Can you work these out from the model? Positions are in its coordinate system, mm. A direction names the side the tool comes from. Coordinates: 2 decimals unless noted, no trailing zeros. Write each loop counter-clockwise with the first axis right and the second up, starting at its lowest first coordinate (ties: lowest second). Pieces come first, ordered by that corner, then holes. Notation, with made-up numbers: (-26.75, 79) - (-2.75, 79) arc R10 cw to (-2.75, 84) - close; hole circle Ø8 at (7.5, 52). An arc over 180 degrees is marked (long way). One line per question, with ' | ' between items. Start each with the question number.
from build123d import *

# Parameters (mm, degrees)
F0_R     = 25
F0_R_2   = 15
F1_DEPTH = 28
F2_DEPTH = 116
F3_DEPTH = 28.5
F4_DEPTH = 50.8


with BuildPart() as f1:
    # F0 (on Top) → F1 (new body)
    with BuildSketch(Plane.XY):
        with BuildLine():
            Line((0, -44.5), (44.5, -44.5))
            Line((44.5, -44.5), (44.5, 0))
            ThreePointArc((44.5, 0), (31.466252, -31.466252), (0, -44.5))
        make_face()
        with BuildLine():
            Line((-44.5, -44.5), (0, -44.5))
            ThreePointArc((0, -44.5), (-31.466252, -31.466252), (-44.5, 0))
            Line((-44.5, 0), (-44.5, -44.5))
        make_face()
        with BuildLine():
            ThreePointArc((0, 44.5), (31.466252, 31.466252), (44.5, 0))
            Line((44.5, 0), (44.5, 44.5))
            Line((44.5, 44.5), (0, 44.5))
        make_face()
        with BuildLine():
            Line((-44.5, 44.5), (-44.5, 0))
            ThreePointArc((-44.5, 0), (-31.466252, 31.466252), (0, 44.5))
            Line((0, 44.5), (-44.5, 44.5))
        make_face()
        Circle(F0_R)
        Circle(F0_R_2, mode=Mode.SUBTRACT)
    extrude(amount=F1_DEPTH)

    # F0 (on Top) → F2 (join)
    with BuildSketch(Plane.XY):
        with BuildLine():
            ThreePointArc((-44.5, 0), (-31.466252, -31.466252), (0, -44.5))
            ThreePointArc((0, -44.5), (31.466252, -31.466252), (44.5, 0))
            ThreePointArc((44.5, 0), (31.466252, 31.466252), (0, 44.5))
            ThreePointArc((0, 44.5), (-31.466252, 31.466252), (-44.5, 0))
        make_face()
        Circle(F0_R, mode=Mode.SUBTRACT)
        Circle(F0_R)
        Circle(F0_R_2, mode=Mode.SUBTRACT)
        Circle(F0_R_2)
    extrude(amount=F2_DEPTH)

    # F0 (on Top) → F3 (join)
    with BuildSketch(Plane.XY):
        Circle(F0_R)
        Circle(F0_R_2, mode=Mode.SUBTRACT)
    extrude(amount=-F3_DEPTH)

    # F0 (on Top) → F4 (join)
    with BuildSketch(Plane.XY):
        Circle(F0_R_2)
    extrude(amount=-F4_DEPTH)


solid = f1.part
(1) If I drill on probe 1 along Z at (x, y) = (-18, 31.5); probe 2 along Z at (x, y) = (16, 10.5); probe 3 along Y at (x, z) = (-1, 49), over which ranges is the centre line in solid material (lowest first)?
(2) Which directions (+Z, -Z, +X, -X, +Y, -Y) give clear straight access to the entire face, cutting with the end or side of a thin tool? Please do faces 1 (the face through (-36, 34, 28)), 2 (the face through (-36, -34, 28)), 3 (the face through (34, 36, 28)), 4 (the face through (11, -11, -28.5)), 5 (the face through (35, -35, 28)).
(3) If we section it at D-D on x = -36.5: List the corners of the cut face in (y, z) for me.
(4) I'm going to push flat-ended pins straight in: pin 1 (3 mm diameter, centred on y = -13, z = 93.5, fed in from +X); pin 2 (1 mm diameter, centred on y = 12.5, z = 84.5, fed in from -X); pin 3 (4 mm diameter, centred on x = 23, y = -14.5, fed in from -Z). Where does each tip first touch, or does it pass through?
(5) If we section it at A-A on x = -19: List the corners of the cut face in (y, z) for me.
(6) If we section it at B-B on y = 33: List the corners of the cut face in (x, z) for me, plus the area to 3 significant figures.
(7) If we section it at C-C on z = 72.5: List the corners of the cut face in (x, y) for me, plus the area to 3 significant figures.
Values:
1) probe 1: 0 to 116 | probe 2: -28.5 to 116 | probe 3: -44.49 to 44.49
2) face 1: +Z, -X, +Y | face 2: +Z, -X, -Y | face 3: +Z, +X, +Y | face 4: -Z | face 5: +Z, +X, -Y
3) outline: (-44.5, 0) - (44.5, 0) - (44.5, 28) - (25.46, 28) - (25.46, 116) - (-25.46, 116) - (-25.46, 28) - (-44.5, 28) - close
4) pin 1: x = 42.99 | pin 2: x = -42.85 | pin 3: z = 0
5) outline: (-44.5, 0) - (-16.25, 0) - (-16.25, -28.5) - (16.25, -28.5) - (16.25, 0) - (44.5, 0) - (44.5, 28) - (40.24, 28) - (40.24, 116) - (-40.24, 116) - (-40.24, 28) - (-44.5, 28) - close
6) outline: (-44.5, 0) - (44.5, 0) - (44.5, 28) - (29.85, 28) - (29.85, 116) - (-29.85, 116) - (-29.85, 28) - (-44.5, 28) - close | area: 7,750 mm2
7) outline: (-44.5, 0) arc R44.5 ccw to (0, -44.5) arc R44.5 ccw to (44.5, 0) arc R44.5 ccw to (0, 44.5) arc R44.5 ccw to start | area: 6,220 mm2
